from build123d import *

# Parameters (mm, degrees)
SKETCH1_W           = 16
SKETCH1_H           = 5
BOSS_EXTRUDE1_DEPTH = 5


with BuildPart() as part:
    # Sketch1 → Boss-Extrude1 (new body)
    with BuildSketch(Plane(origin=(0, 0, 0), x_dir=(1, 0, 0), z_dir=(0, 1, 0))):
        with BuildLine():
            Line((-29.495397245, 40), (29.879619523, 40))
            ThreePointArc((29.879619523, 40), (35.039273824, 40.677009354), (39.849614703, 42.662203251))
            Line((39.849614703, 42.662203251), (62.507501205, 55.691483874))
            ThreePointArc((62.507501205, 55.691483874), (67.503747793, 55.684995753), (70, 51.357034687))
            Line((70, 51.357034687), (70, -51.328756138))
            ThreePointArc((70, -51.328756138), (67.497622519, -55.660254926), (62.495247299, -55.656135704))
            Line((62.495247299, -55.656135704), (40.094909722, -42.690481736))
            ThreePointArc((40.094909722, -42.690481736), (35.262884302, -40.684328056), (30.075898919, -40))
            Line((30.075898919, -40), (-29.621741739, -40))
            ThreePointArc((-29.621741739, -40), (-34.74594239, -40.667577294), (-39.528063042, -42.625743232))
            Line((-39.528063042, -42.625743232), (-62.523419674, -55.737060414))
            ThreePointArc((-62.523419674, -55.737060414), (-67.511682541, -55.716857277), (-70, -51.393496222))
            Line((-70, -51.393496222), (-70, 51.411080519))
            ThreePointArc((-70, 51.411080519), (-67.515524189, 55.732207462), (-62.531144779, 55.759040259))
            Line((-62.531144779, 55.759040259), (-39.370818131, 42.608161042))
            ThreePointArc((-39.370818131, 42.608161042), (-34.602413049, 40.663030497), (-29.495397245, 40))
        make_face()
        Rectangle(SKETCH1_W, SKETCH1_H, mode=Mode.SUBTRACT)
        with Locations((-32, 0)):
            Rectangle(SKETCH1_W, SKETCH1_H, mode=Mode.SUBTRACT)
        with Locations((32, 0)):
            Rectangle(SKETCH1_W, SKETCH1_H, mode=Mode.SUBTRACT)
    extrude(amount=BOSS_EXTRUDE1_DEPTH)


solid = part.part
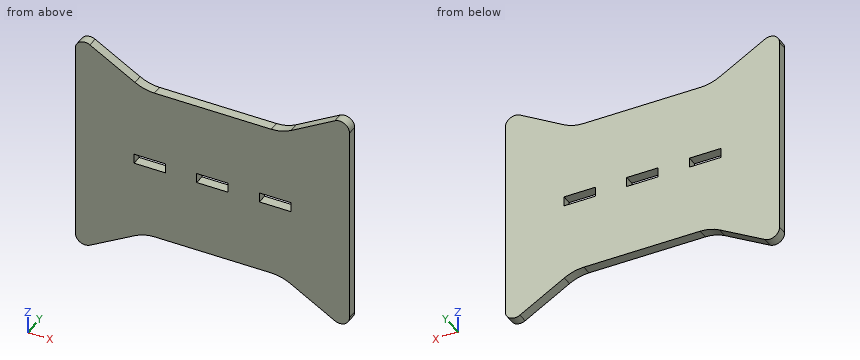
Here's how the part is built. I have some questions about the finished solid (model axes, mm). Round coordinates to 2 decimals unless told otherwise and drop trailing zeros. Write each loop counter-clockwise with the first axis right and the second up, starting at its lowest first coordinate (ties: lowest second). Pieces come first, ordered by that corner, then holes.
1. Suppose I cut it at B-B (y = 3.85). List the corners of the cut face in (x, z) for me.
2. Suppose I cut it at A-A (x = -4). List the corners of the cut face in (y, z) for me, and give its area (3 significant figures).
3. Suppose I cut it at D-D (x = 20). List the corners of the cut face in (y, z) for me, and give its area (3 significant figures).
4. Will these pins go through, and if not, where does the flat tip stop? pin 1 Ø1.5 at (x, y) = (-0.5, 1.5) entering from -Z; pin 2 Ø1.5 at (x, y) = (35, 3.5) entering from +Z; pin 3 Ø2.5 at (x, y) = (1, 2) entering from +Z.
5. Suppose I cut it at C-C (z = 46). List the corners of the cut face in (x, y) for me.
6. I need wall thicknesses on L1, parallel to Z at x = 11, y = 4.4; L2, parallel to Z at x = 31.5, y = 4.85; L3, parallel to Z at x = 37.5, y = 1.75. Which ranges of each line are inside material? Lowest first, please.
Answer sheet:
1. outline: (-70, -51.41) arc R5 ccw to (-62.53, -55.76) - (-39.37, -42.61) arc R20 cw to (-29.5, -40) - (29.88, -40) arc R20 cw to (39.85, -42.66) - (62.51, -55.69) arc R5 ccw to (70, -51.36) - (70, 51.33) arc R5 ccw to (62.5, 55.66) - (40.09, 42.69) arc R20 cw to (30.08, 40) - (-29.62, 40) arc R20 cw to (-39.53, 42.63) - (-62.52, 55.74) arc R5 ccw to (-70, 51.39) - close; hole (-40, -2.5) - (-24, -2.5) - (-24, 2.5) - (-40, 2.5) - close; hole (-8, -2.5) - (8, -2.5) - (8, 2.5) - (-8, 2.5) - close; hole (24, -2.5) - (40, -2.5) - (40, 2.5) - (24, 2.5) - close
2. outline: (0, -40) - (5, -40) - (5, -2.5) - (0, -2.5) - close; (0, 2.5) - (5, 2.5) - (5, 40) - (0, 40) - close
2. area: 375 mm2
3. outline: (0, -40) - (5, -40) - (5, 40) - (0, 40) - close
3. area: 400 mm2
4. pin 1: stops at z = -40
4. pin 2: stops at z = 40.82
4. pin 3: stops at z = 40
5. outline: (-70, 0) - (-45.45, 0) - (-45.45, 5) - (-70, 5) - close; (45.81, 0) - (70, 0) - (70, 5) - (45.81, 5) - close
6. L1: z = -40 to 40
6. L2: z = -40.07 to -2.5, 2.5 to 40.05
6. L3: z = -41.51 to -2.5, 2.5 to 41.43
